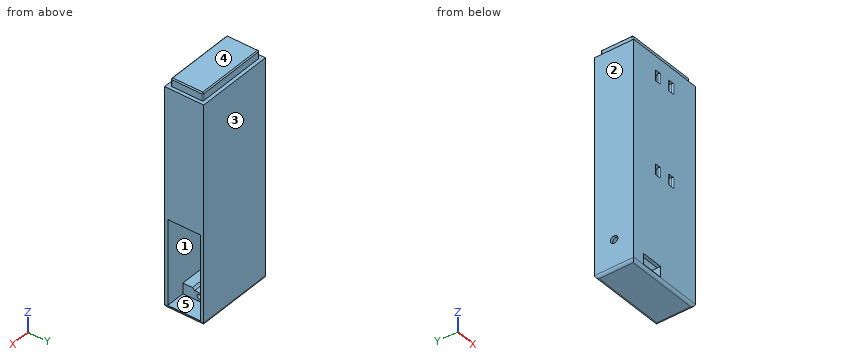
```python
from build123d import *
from OCP.BRepFilletAPI import BRepFilletAPI_MakeChamfer

# Parameters (mm, degrees)
IZIM1_W                     = 29.7
IZIM1_H                     = 14.8
Y_KSEKLIK_EKSTR_ZYON1_DEPTH = 82.2
IZIM2_W                     = 32
IZIM2_H                     = 12.4
KES_EKSTR_ZYON1_DEPTH       = 25
Y_KSEKLIK_EKSTR_ZYON2_START = -7.3
IZIM3_W                     = 4
IZIM3_H                     = 12.4
IZIM3_R                     = 0.85
Y_KSEKLIK_EKSTR_ZYON2_DEPTH = 7
Y_KSEKLIK_EKSTR_ZYON3_START = -0.2
IZIM4_R                     = 0.85
Y_KSEKLIK_EKSTR_ZYON3_DEPTH = 0.2
PAH1_SIZE                   = 3.579571669
PAH1_SIZE_2                 = 6.2
KES_EKSTR_ZYON2_DEPTH       = 3.2
KES_EKSTR_ZYON2_DEPTH_BACK  = 85.630505729
IZIM5_W                     = 8.2
IZIM5_H                     = 4
RADYUS1_R                   = 1
IZIM7_R                     = 1.4
KES_EKSTR_ZYON3_DEPTH       = 87.235723456
IZIM8_W                     = 27.1
IZIM8_H                     = 12.2
Y_KSEKLIK_EKSTR_ZYON4_DEPTH = 3
RADYUS2_R                   = 0.4
IZIM9_W                     = 1.5
IZIM9_H                     = 4
L_O_ALTMA1_COUNT            = 2
L_O_ALTMA1_PITCH            = 35
RADYUS3_R                   = 0.5
KES_EKSTR_ZYON4_REACH       = 90.406
IZIM10_W                    = 0.8
IZIM10_H                    = 3.2
PAH3_SIZE                   = 1
PAH4_SIZE                   = 0.4
KES_EKSTR_ZYON5_DEPTH       = 3.7


# Some blends are built 0.0001 mm under size
with BuildPart() as part:
    # Çizim1 → Yükseklik-Ekstrüzyon1 (new body)
    with BuildSketch(Plane.XY):
        Rectangle(IZIM1_W, IZIM1_H)
    extrude(amount=Y_KSEKLIK_EKSTR_ZYON1_DEPTH)

    # Çizim2 → Kes-Ekstrüzyon1 (cut)
    with BuildSketch(Plane(origin=(14.85, 0, 0), x_dir=(0, 0, -1), z_dir=(1, 0, 0))):
        with Locations((-17.2, 0)):
            Rectangle(IZIM2_W, IZIM2_H)
    extrude(amount=-KES_EKSTR_ZYON1_DEPTH, mode=Mode.SUBTRACT)

    # Çizim3 → Yükseklik-Ekstrüzyon2 (add)
    # profile 1 of 2: a face of its own
    with BuildSketch(Plane(origin=(14.85, 0, 0), x_dir=(0, 0, -1), z_dir=(1, 0, 0)).offset(Y_KSEKLIK_EKSTR_ZYON2_START)):
        with Locations((-31.2, 0)):
            Rectangle(IZIM3_W, IZIM3_H)
        with Locations((-31.45, 0)):
            Circle(IZIM3_R, mode=Mode.SUBTRACT)
    # profile 2 of 2: a face of its own
    with BuildSketch(Plane(origin=(14.85, 0, 0), x_dir=(0, 0, -1), z_dir=(1, 0, 0)).offset(Y_KSEKLIK_EKSTR_ZYON2_START)):
        with Locations((-3.2, 0)):
            Rectangle(IZIM3_W, IZIM3_H)
        with Locations(Location((-2.95, 0, 0), (0, 0, 180))):
            Circle(IZIM3_R, mode=Mode.SUBTRACT)
    extrude(amount=-Y_KSEKLIK_EKSTR_ZYON2_DEPTH)

    # Çizim4 → Yükseklik-Ekstrüzyon3 (add)
    with BuildSketch(Plane.ZY.offset(-0.55).offset(Y_KSEKLIK_EKSTR_ZYON3_START)):
        with Locations(Location((31.45, 0, 0), (0, 0, 180))):
            Circle(IZIM4_R)
        with Locations((2.95, 0)):
            Circle(IZIM4_R)
    extrude(amount=Y_KSEKLIK_EKSTR_ZYON3_DEPTH)

    # Pah1
    pah1_edges_1 = [part.edges().sort_by_distance(p)[0] for p in [
        (0.55, -6.2, 3.2),
    ]]
    pah1_side_1 = [part.faces().sort_by_distance(p)[0] for p in [
        (0.478408567, -6.2, 3.2),
    ]]
    pah1_edges_2 = [part.edges().sort_by_distance(p)[0] for p in [
        (0.55, 6.2, 3.2),
    ]]
    pah1_side_2 = [part.faces().sort_by_distance(p)[0] for p in [
        (0.478408567, 6.2, 3.2),
    ]]
    pah1_edges_3 = [part.edges().sort_by_distance(p)[0] for p in [
        (0.55, -6.2, 31.2),
    ]]
    pah1_side_3 = [part.faces().sort_by_distance(p)[0] for p in [
        (0.478408567, -6.2, 31.2),
    ]]
    pah1_edges_4 = [part.edges().sort_by_distance(p)[0] for p in [
        (0.55, 6.2, 31.2),
    ]]
    pah1_side_4 = [part.faces().sort_by_distance(p)[0] for p in [
        (0.478408567, 6.2, 31.2),
    ]]
    pah1 = BRepFilletAPI_MakeChamfer(part.part.solid().wrapped)
    for e in pah1_edges_1:
        pah1.Add(PAH1_SIZE - 0.0001, PAH1_SIZE_2 - 0.0001, e.wrapped, pah1_side_1[0].wrapped)
    for e in pah1_edges_2:
        pah1.Add(PAH1_SIZE - 0.0001, PAH1_SIZE_2 - 0.0001, e.wrapped, pah1_side_2[0].wrapped)
    for e in pah1_edges_3:
        pah1.Add(PAH1_SIZE - 0.0001, PAH1_SIZE_2 - 0.0001, e.wrapped, pah1_side_3[0].wrapped)
    for e in pah1_edges_4:
        pah1.Add(PAH1_SIZE - 0.0001, PAH1_SIZE_2 - 0.0001, e.wrapped, pah1_side_4[0].wrapped)
    add(Compound.cast(pah1.Shape()), mode=Mode.REPLACE)  # a hair under: the kernel refuses the full size

    # Çizim5 → Kes-Ekstrüzyon2 (cut, two sides: drawn at the far end of the back side and taken through both)
    with BuildSketch(Plane(origin=(0, -6.2, 0), x_dir=(1, 0, 0), z_dir=(0, 1, 0)).offset(-KES_EKSTR_ZYON2_DEPTH_BACK)):
        with Locations((-6.05, -3.2)):
            Rectangle(IZIM5_W, IZIM5_H)
    extrude(amount=KES_EKSTR_ZYON2_DEPTH + KES_EKSTR_ZYON2_DEPTH_BACK, mode=Mode.SUBTRACT)

    # Radyus1
    radyus1_edges = [part.edges().sort_by_distance(p)[0] for p in [
        (0, -7.4, 0),
        (-14.85, 0, 0),
        (0, 7.4, 0),
        (14.85, 0, 0),
    ]]
    fillet(radyus1_edges, radius=RADYUS1_R)

    # Çizim7 → Kes-Ekstrüzyon3 (cut, through all)
    with BuildSketch(Plane(origin=(-10.15, 0, 0), x_dir=(0, 0, -1), z_dir=(1, 0, 0))):
        with Locations((-11, 0)):
            Circle(IZIM7_R)
    extrude(amount=-KES_EKSTR_ZYON3_DEPTH, mode=Mode.SUBTRACT)

    # Çizim8 → Yükseklik-Ekstrüzyon4 (add)
    with BuildSketch(Plane.XY.offset(82.2)):
        Rectangle(IZIM8_W, IZIM8_H)
    extrude(amount=Y_KSEKLIK_EKSTR_ZYON4_DEPTH)

    # Radyus2
    radyus2_edges = [part.edges().sort_by_distance(p)[0] for p in [
        (13.55, -6.1, 83.7),
        (13.55, 6.1, 83.7),
        (-13.55, 6.1, 83.7),
        (-13.55, -6.1, 83.7),
    ]]
    fillet(radyus2_edges, radius=RADYUS2_R)

    # Çizim9 → Kes-Döndür1 (revolve, cut)
    with BuildSketch(Plane.XZ.offset(7.4)):
        with Locations((3.25, 40)):
            Rectangle(IZIM9_W, IZIM9_H)
    kes_d_nd_r1 = revolve(axis=Axis((0, -7.4, 0), (0, 0, 1)), mode=Mode.SUBTRACT)

    # LÇoğaltma1: Kes-Döndür1 ×2
    with Locations(*[(0, 0, i * L_O_ALTMA1_PITCH) for i in range(1, L_O_ALTMA1_COUNT)]):
        add(kes_d_nd_r1, mode=Mode.SUBTRACT)

    # Radyus3
    radyus3_edges = [part.edges().sort_by_distance(p)[0] for p in [
        (2.5, -7.4, 40),
        (4, -7.4, 40),
        (-2.5, -7.4, 40),
        (-4, -7.4, 40),
        (4, -7.4, 75),
        (-4, -7.4, 75),
        (2.5, -7.4, 75),
        (-2.5, -7.4, 75),
    ]]
    fillet(radyus3_edges, radius=RADYUS3_R)

    # Çizim10 → Kes-Ekstrüzyon4 (cut, up to next)
    with BuildSketch(Plane(origin=(7.55, 0, 0), x_dir=(0, 0, -1), z_dir=(1, 0, 0)), mode=Mode.PRIVATE) as kes_ekstr_zyon4_sk1:
        with Locations((-4.8, 0)):
            Rectangle(IZIM10_W, IZIM10_H)
    kes_ekstr_zyon4_tool1 = extrude(kes_ekstr_zyon4_sk1.sketch, amount=-KES_EKSTR_ZYON4_REACH, mode=Mode.PRIVATE) & part.part
    add(kes_ekstr_zyon4_tool1.solids().sort_by_distance((7.55, 0, 4.8))[0], mode=Mode.SUBTRACT)

    # Pah3
    # the kernel refuses this chamfer: 1 mm, written as the material it takes off along each edge
    with BuildSketch(Plane(origin=(10.121682988, -1.6, 5.2), x_dir=(0, -0.9996219169112968, 0.027495876610586473), z_dir=(-1, 0, 0))) as pah3_piece_1_section:
        Polygon((PAH3_SIZE * 0.999621916911, -PAH3_SIZE * 0.0274958766106), (-PAH3_SIZE * 0.0274958766106, -PAH3_SIZE * 0.999621916911), (0, 0), align=None)
    pah3_piece_1 = extrude(amount=13.067057765, mode=Mode.PRIVATE)
    pah3_piece_1 = split(pah3_piece_1, bisect_by=Plane(origin=(3.588154105, -1.945718412, 4.4), z_dir=(0, 0, 1)), keep=Keep.TOP, mode=Mode.PRIVATE)
    add(pah3_piece_1, mode=Mode.SUBTRACT)
    with BuildSketch(Plane(origin=(10.121682988, 1.6, 5.2), x_dir=(0, 0.9996219169112968, 0.027495876610586487), z_dir=(-1, 0, 0))) as pah3_piece_2_section:
        Polygon((PAH3_SIZE * 0.999621916911, PAH3_SIZE * 0.0274958766106), (-PAH3_SIZE * 0.0274958766106, PAH3_SIZE * 0.999621916911), (0, 0), align=None)
    pah3_piece_2 = extrude(amount=13.067057765, mode=Mode.PRIVATE)
    pah3_piece_2 = split(pah3_piece_2, bisect_by=Plane(origin=(3.588154105, 1.945718412, 4.4), z_dir=(0, 0, 1)), keep=Keep.TOP, mode=Mode.PRIVATE)
    add(pah3_piece_2, mode=Mode.SUBTRACT)

    # Pah4
    pah4_edges = [part.edges().sort_by_distance(p)[0] for p in [
        (13.55, 0, 85.2),
        (0, -6.1, 85.2),
        (0, 6.1, 85.2),
        (-13.55, 0, 85.2),
        (-13.432842712, 5.982842712, 85.2),
        (13.432842712, 5.982842712, 85.2),
        (-13.432842712, -5.982842712, 85.2),
        (13.432842712, -5.982842712, 85.2),
    ]]
    chamfer(pah4_edges, length=PAH4_SIZE)

    # Çizim12 → Kes-Ekstrüzyon5 (cut)
    with BuildSketch(Plane(origin=(-10.15, 0, 0), x_dir=(0, 0, -1), z_dir=(1, 0, 0))):
        Polygon((-7.766838493, 0), (-9.383419246, 2.8), (-12.616580754, 2.8), (-14.233161507, 0), (-12.616580754, -2.8), (-9.383419246, -2.8), align=None)
    extrude(amount=-KES_EKSTR_ZYON5_DEPTH, mode=Mode.SUBTRACT)


solid = part.part
```
Verification items for the finished model (mm, model axes). Face numbers are marked on the shaded views. A direction names the side the tool comes from. Coordinates: 2 decimals unless noted, no trailing zeros. Loops run counter-clockwise (first coordinate to the right, second up) from the corner with the lowest first, then second, coordinate; pieces in that order, holes last. Notation, with made-up numbers: (-32.75, 4) - (8.25, 4) arc R8 ccw to (8.25, 9) - close; hole circle Ø11 at (22, 22). An arc over 180 degrees is marked (long way). Answer as a JSON object with one key per item and string values.
(1) Cross-section at C-C, the plane x = -7.5. Record the boundary of the cut face in (y, z).
Response:
{"outline": "(-7.4, 1) arc R1 ccw to (-6.4, 0) - (6.4, 0) arc R1 ccw to (7.4, 1) - (7.4, 82.2) - (6.1, 82.2) - (6.1, 84.8) - (5.7, 85.2) - (-5.7, 85.2) - (-6.1, 84.8) - (-6.1, 82.2) - (-7.4, 82.2) - (-7.4, 5.2) - (-6.2, 5.2) - (-6.2, 33.2) - (6.2, 33.2) - (6.2, 1.2) - (-7.4, 1.2) - close"}
(2) Mould release check, pull along Y, two halves, no side actions. Record for the marked faces 1, 2 and 3: pulls with the +Y half, pulls with the -Y half, needs draft (parallel to the pull), parting line crosses it, or undercut.
Response:
{"face 1": "undercut", "face 2": "needs draft", "face 3": "pulls with the +Y half"}
(3) Cross-section at A-A, the plane z = 11. Record the boundary of the cut face in (x, y), then the cut area to 3 significant figures.
Response:
{"outline": "(-14.85, -7.4) - (14.85, -7.4) - (14.85, -6.2) - (-10.15, -6.2) - (-10.15, -2.8) - (-13.85, -2.8) - (-13.85, -1.4) - (-14.85, -1.4) - close; (-14.85, 1.4) - (-13.85, 1.4) - (-13.85, 2.8) - (-10.15, 2.8) - (-10.15, 6.2) - (14.85, 6.2) - (14.85, 7.4) - (-14.85, 7.4) - close", "area": "106 mm²"}
(4) Go/stop test with flat-tipped pins: pin 1 Ø4 at (y, z) = (-2, 10) entering from +X; pin 2 Ø2 at (y, z) = (0, 84) entering from -X; pin 3 Ø1.9 at (y, z) = (0, 31.5) entering from +X. Record where each tip stops, or that it passes through.
Response:
{"pin 1": "stops at x = -10.15", "pin 2": "stops at x = -13.55", "pin 3": "stops at x = 7.55"}
(5) Scan lines: line 1 along Z through (x, y) = (2.5, 0); line 2 along Y through (x, z) = (4.5, 2.95); line 3 along Z through (x, y) = (1.75, 5.25). Record each from-to range of solid material in increasing order.
Response:
{"line 1": "z = 0 to 2.1, 3.8 to 4.4, 29.2 to 30.6, 32.3 to 85.2", "line 2": "y = -7.4 to -0.85, 0.85 to 7.4", "line 3": "z = 0 to 5.2, 29.2 to 85.2"}
(6) Cross-section at B-B, the plane x = 9.5. Record the boundary of the cut face in (y, z).
Response:
{"outline": "(-7.4, 1) arc R1 ccw to (-6.4, 0) - (6.4, 0) arc R1 ccw to (7.4, 1) - (7.4, 82.2) - (6.1, 82.2) - (6.1, 84.8) - (5.7, 85.2) - (-5.7, 85.2) - (-6.1, 84.8) - (-6.1, 82.2) - (-7.4, 82.2) - close; hole (-6.2, 1.2) - (6.2, 1.2) - (6.2, 33.2) - (-6.2, 33.2) - close"}
(7) Access from +Z, -Z, +X, -X, +Y, -Y to the whole of each face (thin tool, end or side, straight path). Record for the marked faces 4 and 5.
Response:
{"face 4": "+Z, +X, -X, +Y, -Y", "face 5": "+X"}
(8) Cross-section at D-D, the plane z = 26. Record the boundary of the cut face in (x, y), then the cut area to 3 significant figures.
Response:
{"outline": "(-14.85, -7.4) - (14.85, -7.4) - (14.85, -6.2) - (-10.15, -6.2) - (-10.15, 6.2) - (14.85, 6.2) - (14.85, 7.4) - (-14.85, 7.4) - close", "area": "130 mm²"}
